from build123d import *

# Parameters (mm, degrees)
SKETCH1_R           = 3.025
SKETCH1_R_2         = 2.025
BOSS_EXTRUDE1_DEPTH = 15
BOSS_EXTRUDE2_START = 6
SKETCH1_2_R         = 3.025
BOSS_EXTRUDE2_DEPTH = 9
SKETCH2_R           = 2.65
CUT_EXTRUDE1_DEPTH  = 3


with BuildPart() as part:
    # Sketch1 → Boss-Extrude1 (new body)
    with BuildSketch(Plane.XY):
        Polygon((66.489922843, -72.31585339), (69.489922843, -72.31585339), (69.489922843, -92.31585339), (89.489922843, -92.31585339), (89.489922843, -95.31585339), (66.489922843, -95.31585339), (49.489922843, -87.66585339), (49.489922843, -73.16585339), align=None)
        with Locations((56.489922843, -77.31585339)):
            Circle(SKETCH1_R, mode=Mode.SUBTRACT)
        with Locations((53.489922843, -84.31585339)):
            Circle(SKETCH1_R_2, mode=Mode.SUBTRACT)
        with Locations((59.489922843, -84.31585339)):
            Circle(SKETCH1_R_2, mode=Mode.SUBTRACT)
    extrude(amount=BOSS_EXTRUDE1_DEPTH)

    # Sketch1<2> → Boss-Extrude2 (add)
    with BuildSketch(Plane.XY.offset(BOSS_EXTRUDE2_START)):
        with Locations((56.489922843, -77.31585339)):
            Circle(SKETCH1_2_R)
    extrude(amount=BOSS_EXTRUDE2_DEPTH)

    # Sketch2 → Cut-Extrude1 (cut)
    with BuildSketch(Plane.XZ.offset(95.31585339)):
        with Locations((79.489922843, 7.5)):
            Circle(SKETCH2_R)
    extrude(amount=-CUT_EXTRUDE1_DEPTH, mode=Mode.SUBTRACT)


solid = part.part
Check sheet for the modelled part. Datum: model origin and axes. Units: mm. A direction names the side the tool comes from. Give positions to 0.01 mm unless a question says otherwise; leave off trailing zeros. Loops run counter-clockwise (first coordinate to the right, second up) from the corner with the lowest first, then second, coordinate; pieces in that order, holes last. Notation, with made-up numbers: M -29,17.5 L -4,17.5 A17 ccw -4,43.5 Z; hole C -13.75,-13.75 d2. An arc over 180 degrees is marked long. Answer as a JSON object with one key per item and string values. Group by question number.
Q1. Cross-section at C-C on z = 11.5. Record the cut outline in (x, y) (3 decimals), then the cut area to 3 significant figures.
Q2. Cross-section at A-A on z = 6.5. Record the cut outline in (x, y) (3 decimals), then the cut area to 3 significant figures.
Q3. Release check for a two-part mould opening along X. For faces 4 (the cylindrical face through (51.883, -85.548, 7.395)), 5 (the flat face through (68, -72.316, 7)), 6 (the flat face through (57.871, -72.747, 7.395)), 7 (the flat face through (56, -77, 6)) record: released by +X, released by -X, zero draft, split by the parting line, or undercut.
Q4. Cross-section at D-D on x = 86. Record the cut outline in (y, z).
Q5. Material ranges on line 1 along X through (y, z) = (-86, 5.25); line 2 along Y through (x, z) = (74, 12.25); line 3 along Y through (x, z) = (52, 12.5), recorded low to high. Write a range as [from, to].
Q6. Go/stop test with flat-tipped pins: P1, Ø8.5, axis at x = 79.49, z = 7.5, coming from the +Y side; P2, Ø3.5, axis at x = 53.49, y = -84.32, coming from the -Z side; P3, Ø1, axis at y = -78, z = 12.5, coming from the +X side; P4, Ø5, axis at x = 55.5, z = 13, coming from the -Y side. Record where each tip stops, or that it passes through.
Q7. Access from +Z, -Z, +X, -X, +Y, -Y to the whole of each face (thin tool, end or side, straight path). Record for faces 1 (the cylindrical face through (57.886, -80, 2.958)), 2 (the flat face through (89.49, -94, 7)), 3 (the flat face through (77, -92.316, 6)).
Q8. Cross-section at B-B on y = -84.75. Record the cut outline in (x, z).
Evaluation:
{
 "1": {"outline": "M 49.49,-87.666 L 66.49,-95.316 L 89.49,-95.316 L 89.49,-92.316 L 69.49,-92.316 L 69.49,-72.316 L 66.49,-72.316 L 49.49,-73.166 Z; hole C 53.49,-84.316 d4.05; hole C 59.49,-84.316 d4.05", "area": "422 mm2"},
 "2": {"outline": "M 49.49,-87.666 L 66.49,-95.316 L 77.036,-95.316 L 77.036,-92.316 L 69.49,-92.316 L 69.49,-72.316 L 66.49,-72.316 L 49.49,-73.166 Z; M 81.944,-95.316 L 89.49,-95.316 L 89.49,-92.316 L 81.944,-92.316 Z; hole C 53.49,-84.316 d4.05; hole C 59.49,-84.316 d4.05", "area": "407 mm2"},
 "3": {"face 4": "undercut", "face 5": "zero draft", "face 6": "released by -X", "face 7": "undercut"},
 "4": {"outline": "M -95.32,0 L -92.32,0 L -92.32,15 L -95.32,15 Z"},
 "5": {"line 1": "x = [49.49, 52.37], [54.61, 58.37], [60.61, 69.49]", "line 2": "y = [-95.32, -92.32]", "line 3": "y = [-88.8, -85.69], [-82.94, -73.04]"},
 "6": {"P1": "stops at y = -92.32", "P2": "passes through", "P3": "stops at x = 69.49", "P4": "stops at y = -91.5"},
 "7": {"face 1": "-Z", "face 2": "+Z, -Z, +X, +Y, -Y", "face 3": "+Z, -Z, +X, +Y"},
 "8": {"outline": "M 49.49,0 L 51.51,0 L 51.51,15 L 49.49,15 Z; M 55.47,0 L 57.51,0 L 57.51,15 L 55.47,15 Z; M 61.47,0 L 69.49,0 L 69.49,15 L 61.47,15 Z"}
}
